Job drawing, mm, ordinate dimensions from the low corner. One solid piece. A direction names the side the tool comes from. Round coordinates to 2 decimals unless told otherwise and drop trailing zeros. Loops run counter-clockwise (first coordinate to the right, second up) from the corner with the lowest first, then second, coordinate; pieces in that order, holes last. Notation, with made-up numbers: M 62,78.25 L 77,78.25 A7 ccw 77,91.25 Z; hole C 62.25,17.25 d1. An arc over 180 degrees is marked long. Use a Markdown table: item, result. Add a question column.
(1) Wall check: L1, parallel to X at y = 38, z = 8.5; L2, parallel to Z at x = 46, y = 15.5; L3, parallel to X at y = 32.5, z = 54 (1 decimal). Give the ranges that are in metal, low to high.
(2) Flat gauge pins, fed straight in: P1, Ø4.5, axis at x = 46.5, z = 57, coming from the +Y side; P2, Ø8, axis at x = 52, z = 45.5, coming from the +Y side. Where does each tip first touch, or does it go through?
(3) Which spindle directions (+Z, -Z, +X, -X, +Y, -Y) get a long thin tool onto all of the face, cutting with end or side? Do the marked faces 4 and 5. Say none if no direction does.
(4) Band-saw the part on C-C, the plane z = 30.5. Write the cut outline in (x, y), and give its area (3 significant figures).
(5) Two-plate mould, pull along X, no slides. Class the marked faces 1, 2 and 3: released by +X, released by -X, zero draft, split by the parting line, or undercut.
(6) Band-saw the part on B-B, the plane y = 23. Write the cut outline in (x, z), and give its area (3 significant figures).
(7) Band-saw the part on D-D, the plane z = 55. Write the cut outline in (x, y) (1 decimal), and give its area (3 significant figures).
(8) Band-saw the part on A-A, the plane x = 31. Write the cut outline in (y, z), and give its area (3 significant figures).
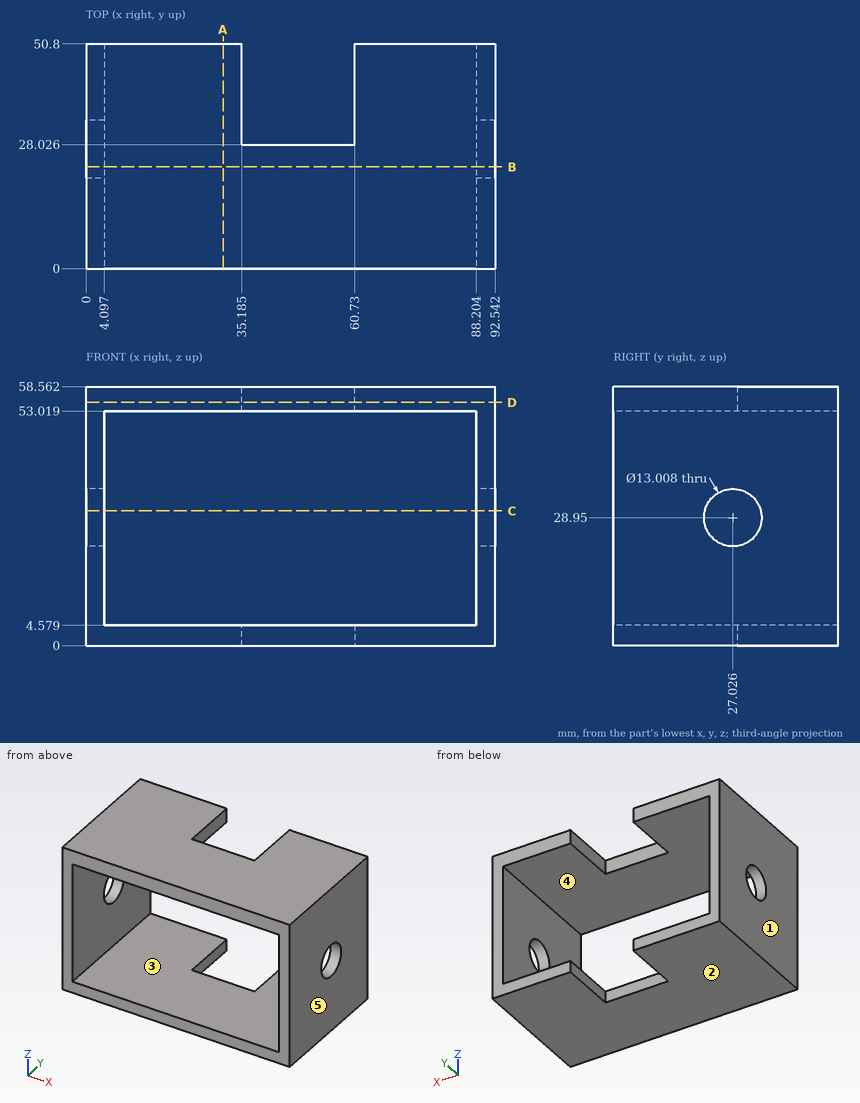
Return value:
| question | item | result |
|---|---|---|
| 1 | L1 | 0 to 4.1, 88.2 to 92.54 |
| 1 | L2 | 0 to 4.58, 53.02 to 58.56 |
| 1 | L3 | 0 to 35.2, 60.7 to 92.5 |
| 2 | P1 | y = 28.03 |
| 2 | P2 | through |
| 3 | face 4 | +Y, -Y |
| 3 | face 5 | +Z, -Z, +X, +Y, -Y |
| 4 | outline | M 0,0 L 4.1,0 L 4.1,20.71 L 0,20.71 Z; M 0,33.34 L 4.1,33.34 L 4.1,50.8 L 0,50.8 Z; M 88.2,0 L 92.54,0 L 92.54,20.71 L 88.2,20.71 Z; M 88.2,33.34 L 92.54,33.34 L 92.54,50.8 L 88.2,50.8 Z |
| 4 | area | 322 mm^2 |
| 5 | face 1 | released by -X |
| 5 | face 2 | zero draft |
| 5 | face 3 | undercut |
| 6 | outline | M 0,0 L 92.54,0 L 92.54,23.84 L 88.2,23.84 L 88.2,4.58 L 4.1,4.58 L 4.1,23.84 L 0,23.84 Z; M 0,34.06 L 4.1,34.06 L 4.1,53.02 L 88.2,53.02 L 88.2,34.06 L 92.54,34.06 L 92.54,58.56 L 0,58.56 Z |
| 6 | area | 1,260 mm^2 |
| 7 | outline | M 0,0 L 92.5,0 L 92.5,50.8 L 60.7,50.8 L 60.7,28 L 35.2,28 L 35.2,50.8 L 0,50.8 Z |
| 7 | area | 4,120 mm^2 |
| 8 | outline | M 0,0 L 50.8,0 L 50.8,4.58 L 0,4.58 Z; M 0,53.02 L 50.8,53.02 L 50.8,58.56 L 0,58.56 Z |
| 8 | area | 514 mm^2 |
